```python
from build123d import *

# Parameters (mm, degrees)
BOSS_EXTRUDE1_DEPTH      = 12.5
BOSS_EXTRUDE3_REACH      = 29.026
BOSS_EXTRUDE3_END_RADIUS = 7.8375
SKETCH5_W                = 7
SKETCH5_H                = 2
SKETCH6_R                = 1.5
CUT_EXTRUDE2_DEPTH       = 2
FILLET2_R                = 1
FILLET2_OF_MIRROR2_R     = 1
BOSS_EXTRUDE4_DEPTH      = 1
SKETCH11_W               = 3
SKETCH11_H               = 7.5
CUT_EXTRUDE4_DEPTH       = 40.134350283
FILLET3_R                = 1


with BuildPart() as part:
    # Sketch1 → Boss-Extrude1 (new, symmetric)
    with BuildSketch(Plane.XY):
        with BuildLine():
            Line((-7.821534776, 0.5), (-6.229967897, 0.5))
            ThreePointArc((-6.229967897, 0.5), (0, 6.25), (6.229967897, 0.5))
            Line((6.229967897, 0.5), (7.821534776, 0.5))
            ThreePointArc((7.821534776, 0.5), (0, 7.8375), (-7.821534776, 0.5))
        make_face()
    extrude(amount=BOSS_EXTRUDE1_DEPTH, both=True)

    # Boss-Extrude3: up to this cylinder (the profile starts outside it)
    boss_extrude3_end = Plane(origin=(0, 0, 0), z_dir=(0, 0, -1)) * Cylinder(BOSS_EXTRUDE3_END_RADIUS, 74.727, mode=Mode.PRIVATE)
    # Sketch5 → Boss-Extrude3 (add, up to the surface)
    with BuildSketch(Plane(origin=(14.821534776, 0, 0), x_dir=(0, 0, -1), z_dir=(1, 0, 0)), mode=Mode.PRIVATE) as boss_extrude3_sk1:
        with Locations((0, 1.5)):
            Rectangle(SKETCH5_W, SKETCH5_H)
    boss_extrude3_tool1 = extrude(boss_extrude3_sk1.sketch, amount=-BOSS_EXTRUDE3_REACH, mode=Mode.PRIVATE) - boss_extrude3_end
    boss_extrude3 = boss_extrude3_tool1.solids().sort_by_distance((14.821535, 1.5, 0))[0]
    add(boss_extrude3)

    # Sketch6 → Cut-Extrude2 (cut)
    with BuildSketch(Plane(origin=(0, 2.5, 0), x_dir=(1, 0, 0), z_dir=(0, 1, 0))):
        with Locations(Location((11.321534776, 0, 0), (0, 0, 270))):
            Circle(SKETCH6_R)
    cut_extrude2 = extrude(amount=-CUT_EXTRUDE2_DEPTH, mode=Mode.SUBTRACT)

    # Fillet2
    fillet2_edges = [part.edges().sort_by_distance(p)[0] for p in [
        (14.821534776, 1.5, 3.5),
        (14.821534776, 1.5, -3.5),
        (7.690104358, 1.512845405, -3.5),
        (7.428082273, 2.5, 0),
        (7.690104358, 1.512845405, 3.5),
    ]]
    fillet(fillet2_edges, radius=FILLET2_R)

    # Mirror2: Boss-Extrude3, Cut-Extrude2 across plane
    add(boss_extrude3.mirror(Plane(origin=(0, 0, 0), x_dir=(0, 0, 1), z_dir=(1, 0, 0))))
    add(cut_extrude2.mirror(Plane(origin=(0, 0, 0), x_dir=(0, 0, 1), z_dir=(1, 0, 0))), mode=Mode.SUBTRACT)

    # Fillet2 of Mirror2
    fillet2_of_mirror2_edges = [part.edges().sort_by_distance(p)[0] for p in [
        (-14.821534776, 1.5, 3.5),
        (-14.821534776, 1.5, -3.5),
        (-7.690104358, 1.512845405, -3.5),
        (-7.428082273, 2.5, 0),
        (-7.690104358, 1.512845405, 3.5),
    ]]
    fillet(fillet2_of_mirror2_edges, radius=FILLET2_OF_MIRROR2_R)

    # Sketch8 → Boss-Extrude4 (add, symmetric)
    with BuildSketch(Plane(origin=(0, 0, 0), x_dir=(0, 0, -1), z_dir=(1, 0, 0))):
        Polygon((12.5, 6.25), (15.5, 9.25), (15.5, 7.8375), (22.5, 7.8375), (22.5, 27.8375), (15.5, 27.8375), (15.5, 15.25), (6.5, 6.25), align=None)
    extrude(amount=BOSS_EXTRUDE4_DEPTH, both=True)

    # Sketch11 → Cut-Extrude4 (cut, through all)
    with BuildSketch(Plane(origin=(1, 0, 0), x_dir=(0, 0, -1), z_dir=(1, 0, 0))):
        with BuildLine():
            Line((20.5, 25.3375), (20.5, 18.3375))
            ThreePointArc((20.5, 18.3375), (19, 16.8375), (17.5, 18.3375))
            Line((17.5, 18.3375), (17.5, 25.3375))
            ThreePointArc((17.5, 25.3375), (19, 26.8375), (20.5, 25.3375))
        make_face()
        with Locations((19, 11.5875)):
            Rectangle(SKETCH11_W, SKETCH11_H)
    extrude(amount=-CUT_EXTRUDE4_DEPTH, mode=Mode.SUBTRACT)

    # Fillet3
    fillet3_edges = [part.edges().sort_by_distance(p)[0] for p in [
        (0, 15.25, -15.5),
        (0, 7.8375, -15.5),
        (0, 7.8375, -22.5),
        (0, 27.8375, -22.5),
        (0, 27.8375, -15.5),
        (-7.025751337, 0.5, 12.5),
        (-7.025751337, 0.5, -12.5),
        (7.025751337, 0.5, -12.5),
        (7.025751337, 0.5, 12.5),
    ]]
    fillet(fillet3_edges, radius=FILLET3_R)


solid = part.part
```
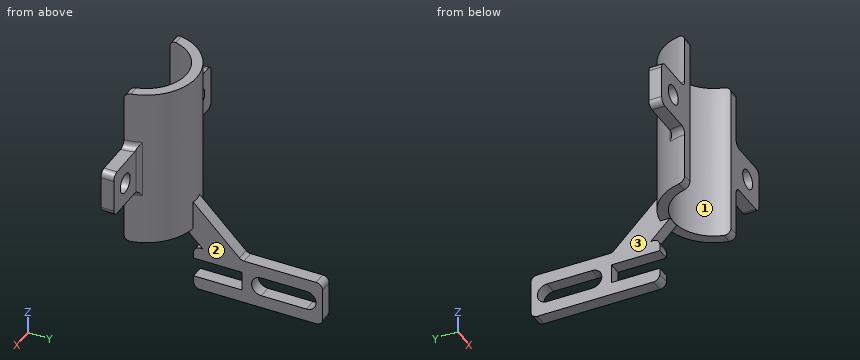
Model file for the job. Use its own axes, mm. Face numbers are marked on the shaded views. Round coordinates to 2 decimals unless told otherwise and drop trailing zeros. Order: outer loops, then holes, each group sorted by start corner. A loop starts at its lowest first (then second) coordinate and runs counter-clockwise, first axis right, second up. Notation, with made-up numbers: (14, 49) -> (22, 49) arc R34 ccw to (22, 82) -> close; hole circle Ø1 at (-34.75, 40.5). An arc over 180 degrees is marked (long way). Use one line per item in the form item = value.
Item 1: Cut at A-A, the plane z = -19. Write the cut outline in (x, y).
Returned:
outline = (-1, 15.34) -> (1, 15.34) -> (1, 16.84) -> (-1, 16.84) -> close; (-1, 26.84) -> (1, 26.84) -> (1, 27.84) -> (-1, 27.84) -> close
Item 2: Flat gauge pins, fed straight in: pin 1 Ø0.6 at (x, y) = (11.5, 2) entering from +Z; pin 2 Ø11.5 at (y, z) = (12, -14) entering from -X; pin 3 Ø8 at (y, z) = (9, -3) entering from -X; pin 4 Ø8 at (x, y) = (-2.5, 10) entering from -Z. Where does each tip first touch, or does it go through?
Returned:
pin_1 = 3.5
pin_2 = -4.45
pin_3 = -6.04
pin_4 = -22.5
Item 3: Drill centre lines: line 1 (X direction, y = 1.7, z = 0); line 2 (X direction, y = 1.4, z = 0); line 3 (X direction, y = 5.5, z = 6). Where is each one in solid material? Low to high.
Returned:
line_1 = -14.82 to -12.82, -9.82 to -6.01, 6.01 to 9.82, 12.82 to 14.82
line_2 = -14.82 to -12.82, -9.82 to -6.09, 6.09 to 9.82, 12.82 to 14.82
line_3 = -5.58 to -2.97, 2.97 to 5.58
Item 4: Cut at C-C, the plane z = 0. Give the number of separate pieces and of enclosed holes in the cut face, and give its area (3 significant figures).
Returned:
separate_pieces = 3
enclosed_holes = 0
area = 50.3 mm^2
Item 5: Cut at B-B, the plane y = 12.5. Write the cut outline in (x, z).
Returned:
outline = (-1, -22.5) -> (1, -22.5) -> (1, -20.5) -> (-1, -20.5) -> close; (-1, -17.5) -> (1, -17.5) -> (1, -12.75) -> (-1, -12.75) -> close
Item 6: Pull direction X, two halves, no side cores. Call the marked faces 1, 2 and 3: released by +X, released by -X, zero draft, split by the parting line, or undercut.
Returned:
face_1 = undercut
face_2 = released by +X
face_3 = released by -X
